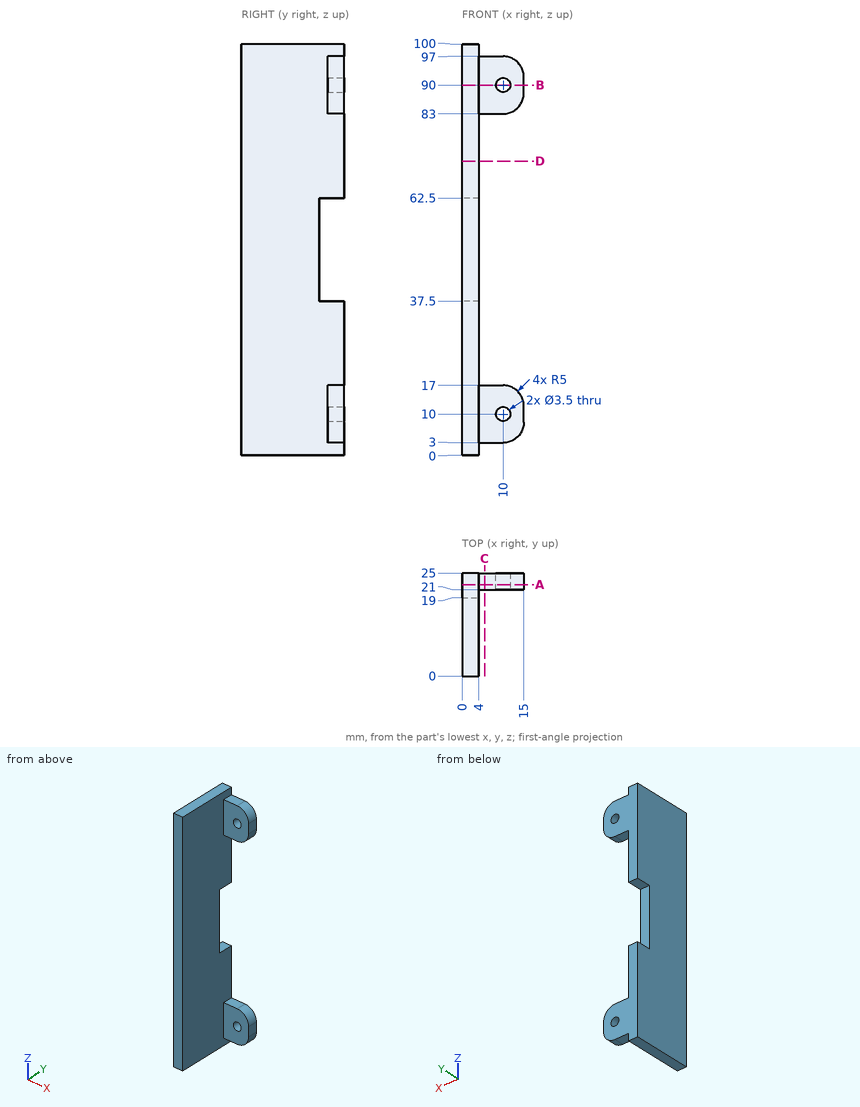
Print and shaded views of the part. All mm, measured from the part's lowest x, y and z. Coordinates: 2 decimals unless noted, no trailing zeros. Order: outer loops, then holes, each group sorted by start corner. A loop starts at its lowest first (then second) coordinate and runs counter-clockwise, first axis right, second up.
(1) Slice it at A-A, the plane y = 22.25. Write the cut outline in (x, z), and give its area (3 significant figures).
Check sheet entries:
outline: (0, 0) - (4, 0) - (4, 3) - (10, 3) arc R5 ccw to (15, 8) - (15, 12) arc R5 ccw to (10, 17) - (4, 17) - (4, 37.5) - (0, 37.5) - close; (0, 62.5) - (4, 62.5) - (4, 83) - (10, 83) arc R5 ccw to (15, 88) - (15, 92) arc R5 ccw to (10, 97) - (4, 97) - (4, 100) - (0, 100) - close; hole circle Ø3.5 at (10, 10); hole circle Ø3.5 at (10, 90)
area: 567 mm2
(2) Slice it at B-B, the plane z = 90. Write the cut outline in (x, y), and give its area (3 significant figures).
Check sheet entries:
outline: (0, 0) - (4, 0) - (4, 21) - (8.25, 21) - (8.25, 25) - (0, 25) - close; (11.75, 21) - (15, 21) - (15, 25) - (11.75, 25) - close
area: 130 mm2
(3) Slice it at D-D, the plane z = 71.5. Write the cut outline in (x, y).
Check sheet entries:
outline: (0, 0) - (4, 0) - (4, 25) - (0, 25) - close
(4) Probe L1, parallel to Z at x = 10, y = 22.2; L2, parallel to X at y = 22.7, z = 10; L3, parallel to X at y = 17.75, z = 51. List the from-to ranges inside material, lowest first.
Check sheet entries:
L1: z = 3 to 8.25, 11.75 to 17, 83 to 88.25, 91.75 to 97
L2: x = 0 to 8.25, 11.75 to 15
L3: x = 0 to 4
(5) Slice it at C-C, the plane x = 5.5. Write the cut outline in (y, z), and give its area (3 significant figures).
Check sheet entries:
outline: (21, 3) - (25, 3) - (25, 17) - (21, 17) - close; (21, 83) - (25, 83) - (25, 97) - (21, 97) - close
area: 112 mm2
(6) Pin check, flat tips, straight feed: pin 1 Ø4.5 at (x, z) = (2, 50.5) entering from +Y; pin 2 Ø5.5 at (x, z) = (7, 8.5) entering from -Y; pin 3 Ø12.5 at (y, z) = (18, 66.5) entering from +X; pin 4 Ø3 at (x, z) = (10, 10) entering from -Y. Stop position of each tip, or through.
Check sheet entries:
pin 1: stops at y = 19
pin 2: stops at y = 21
pin 3: stops at x = 4
pin 4: passes through
